```python
from build123d import *

# Parameters (mm, degrees)
F0_R     = 12.5
F1_DEPTH = 30
F2_R     = 5


with BuildPart() as f1:
    # F0 (on Top) → F1 (new body)
    with BuildSketch(Plane.XY):
        Polygon((102.857415, -70.30526), (77.678429, 72.491864), (-130.231866, 6.937999), (-157.469519, 53.252321), (-141.420811, -20.010486), (51.016164, 22.144119), (63.246589, -47.218068), (32.226125, -9.502765), (-137.142585, -70.30526), align=None)
        with Locations((19.731589, -45.006815)):
            Circle(F0_R, mode=Mode.SUBTRACT)
    extrude(amount=F1_DEPTH)

    # F2
    f2_edges = [f1.edges().sort_by_distance(p)[0] for p in [
        (-130.231866, 6.937999, 15),
        (-157.469519, 53.252321, 15),
        (-141.420811, -20.010486, 15),
        (32.226125, -9.502765, 15),
        (63.246589, -47.218068, 15),
        (51.016164, 22.144119, 15),
        (-137.142585, -70.30526, 15),
        (77.678429, 72.491864, 15),
        (102.857415, -70.30526, 15),
    ]]
    fillet(f2_edges, radius=F2_R)


solid = f1.part
```
Read the model definition and answer for the solid it produces. Units are mm, in the model's axes. A direction names the side the tool comes from. Give positions to 0.01 mm unless a question says otherwise; leave off trailing zeros. Write each loop counter-clockwise with the first axis right and the second up, starting at its lowest first coordinate (ties: lowest second). Pieces come first, ordered by that corner, then holes. Notation, with made-up numbers: (-38.75, -29) -> (20.25, -29) arc R15 cw to (20.25, -18) -> close; hole circle Ø8 at (19.25, -39). An arc over 180 degrees is marked (long way). Answer in a Markdown table with one row per item.
1) Section C-C on z = 13.5 is taken. Give the vertices of the cut face in (x, y) (3 decimals).
Results list:
| item | result |
|---|---|
| outline | (-150.754, 22.595) -> (-142.491, -15.126) arc R5 ccw to (-136.537, -18.941) -> (45.927, 21.029) arc R5 cw to (51.921, 17.013) -> (59.941, -28.473) arc R5 cw to (51.156, -32.518) -> (34.463, -12.222) arc R5 ccw to (28.912, -10.693) -> (-110.106, -60.599) arc R5 ccw to (-108.417, -70.305) -> (96.899, -70.305) arc R5 ccw to (101.823, -64.437) -> (78.668, 66.877) arc R5 ccw to (72.241, 70.777) -> (-126.436, 8.135) arc R5 cw to (-132.249, 10.369) -> (-141.56, 26.2) arc R5 ccw to start; hole circle Ø25 at (19.732, -45.007) |
2) A tool of negligible diameter and unlimited length cuts with its end or side. For faces 1 (the flat face through (-46.582, 0.765, 14.79)), 2 (the flat face through (-25.707, 39.895, 14.79)), 3 (the flat face through (2, -30, 0)), from which of +Z, -Z, +X, -X, +Y, -Y can it reach the whole face along a straight path? Write none if from no direction.
Results list:
| item | result |
|---|---|
| face 1 | +Z, -Z |
| face 2 | +Z, -Z, +Y |
| face 3 | -Z, +X, -X, +Y, -Y |
3) Section A-A on x = -2.5 is taken. Give the vertices of the cut face in (y, z), plus the area to 3 significant figures.
Results list:
| item | result |
|---|---|
| outline | (-70.31, 0) -> (-21.97, 0) -> (-21.97, 30) -> (-70.31, 30) -> close; (10.42, 0) -> (47.21, 0) -> (47.21, 30) -> (10.42, 30) -> close |
| area | 2,550 mm^2 |
4) Determine the mould class of faces 4 (the flat face through (2, -30, 30)), 5 (the flat face through (-7, -70.305, 15)), 6 (the flat face through (42.926, -22.512, 14.79)), 7 (the cylindrical face through (76.39, 70.25, 15.21)) for opening direction Y: released by +Y, released by -Y, zero draft, split by the parting line, or undercut.
Results list:
| item | result |
|---|---|
| face 4 | zero draft |
| face 5 | released by -Y |
| face 6 | undercut |
| face 7 | released by +Y |
5) Each of these flat-tipped pins is pushed along its axis until it touches: pin 1 Ø3 at (y, z) = (-6.5, 9.5) entering from +X; pin 2 Ø10 at (y, z) = (-23.5, 12) entering from +X; pin 3 Ø8 at (x, z) = (-26, 10) entering from +Y; pin 4 Ø15 at (x, y) = (19.73, -45.01) entering from +Z. Where does it stop, or does it pass through?
Results list:
| item | result |
|---|---|
| pin 1 | x = 91.87 |
| pin 2 | x = 95.49 |
| pin 3 | y = 41.06 |
| pin 4 | through |
6) Straight lines are drawn through the part: line 1 (Y direction, x = -44, z = 25.25); line 2 (Y direction, x = -41, z = 20.5); line 3 (Y direction, x = -129, z = 13). For each, find the intervals that lie inside material, in ascending order. Write a range as [from, to].
Results list:
| item | result |
|---|---|
| line 1 | [-70.31, -36.87], [1.33, 34.13] |
| line 2 | [-70.31, -35.79], [1.99, 35.07] |
| line 3 | [-17.29, 8.02] |
7) Section D-D on x = 26.5 is taken. Give the vertices of the cut face in (y, z).
Results list:
| item | result |
|---|---|
| outline | (-70.31, 0) -> (-55.52, 0) -> (-55.52, 30) -> (-70.31, 30) -> close; (-34.5, 0) -> (-11.56, 0) -> (-11.56, 30) -> (-34.5, 30) -> close; (16.77, 0) -> (56.36, 0) -> (56.36, 30) -> (16.77, 30) -> close |
8) Section B-B on y = -23 is taken. Give the vertices of the cut face in (x, z).
Results list:
| item | result |
|---|---|
| outline | (-5.37, 0) -> (43.33, 0) -> (43.33, 30) -> (-5.37, 30) -> close; (58.98, 0) -> (94.52, 0) -> (94.52, 30) -> (58.98, 30) -> close |
